```python
from build123d import *

# Parameters (mm, degrees)
BOSS_EXTRU_1_DEPTH      = 5
ESQUISSE2_W             = 17
ESQUISSE2_H             = 18
ENL_V_MAT_EXTRU_1_DEPTH = 253.408894455
ESQUISSE3_W             = 6
ESQUISSE3_H             = 41
BOSS_EXTRU_2_DEPTH      = 70
ENL_V_MAT_EXTRU_3_DEPTH = 223.904127373
CHANFREIN1_SIZE         = 3
ESQUISSE7_R             = 1.5
ENL_V_MAT_EXTRU_4_DEPTH = 25


# Read off the part's stored shape, not the designer's step: Boss.-Extru.1
with BuildPart() as part:
    # Boss.-Extru.1 outline → Boss.-Extru.1 (new body)
    with BuildSketch(Plane.XY):
        Polygon((0, 25.5), (0, 0), (240, 0), (240, 25.5), (245, 25.5), (245, 40.5), (240, 40.5), (240, 60.5), (122.5, 60.5), (122.5, 39.5), (117.5, 39.5), (117.5, 60.5), (0, 60.5), (0, 40.5), (-5, 40.5), (-5, 25.5), align=None)
    extrude(amount=BOSS_EXTRU_1_DEPTH)

    # Esquisse2 → Enlèv. mat.-Extru.1 (cut, through all)
    with BuildSketch(Plane.XY.offset(5)):
        with Locations((231.5, 9)):
            Rectangle(ESQUISSE2_W, ESQUISSE2_H)
        with Locations((8.5, 9)):
            Rectangle(ESQUISSE2_W, ESQUISSE2_H)
    extrude(amount=-ENL_V_MAT_EXTRU_1_DEPTH, mode=Mode.SUBTRACT)

    # Esquisse3 → Boss.-Extru.2 (add)
    with BuildSketch(Plane.XY.offset(5)):
        with Locations((47, 22.5)):
            Rectangle(ESQUISSE3_W, ESQUISSE3_H)
        with Locations((193, 22.5)):
            Rectangle(ESQUISSE3_W, ESQUISSE3_H)
    extrude(amount=BOSS_EXTRU_2_DEPTH)

    # Esquisse6 → Enlèv. mat.-Extru.3 (cut, through all)
    with BuildSketch(Plane.ZY.offset(-44)):
        Polygon((35, 43), (75, 43), (75, 2), (61, 2), align=None)
    extrude(amount=-ENL_V_MAT_EXTRU_3_DEPTH, mode=Mode.SUBTRACT)

    # Chanfrein1
    chanfrein1_edges = [part.edges().sort_by_distance(p)[0] for p in [
        (120, 0, 0),
    ]]
    chamfer(chanfrein1_edges, length=CHANFREIN1_SIZE)

    # Esquisse7 → Enlèv. mat.-Extru.4 (cut)
    with BuildSketch(Plane.XZ.offset(-2)):
        with Locations(Location((47, 25, 0), (0, 0, 270))):
            Circle(ESQUISSE7_R)
        with Locations(Location((47, 41, 0), (0, 0, 270))):
            Circle(ESQUISSE7_R)
        with Locations(Location((193, 41, 0), (0, 0, 270))):
            Circle(ESQUISSE7_R)
        with Locations(Location((193, 25, 0), (0, 0, 270))):
            Circle(ESQUISSE7_R)
    extrude(amount=-ENL_V_MAT_EXTRU_4_DEPTH, mode=Mode.SUBTRACT)


solid = part.part
```
Build history of the part. All positions in model axes, mm. A direction names the side the tool comes from. Round coordinates to 2 decimals unless told otherwise and drop trailing zeros. Write each loop counter-clockwise with the first axis right and the second up, starting at its lowest first coordinate (ties: lowest second). Pieces come first, ordered by that corner, then holes. Notation, with made-up numbers: (8.5, 39) - (47.5, 39) arc R26 cw to (47.5, 77) - close; hole circle Ø2 at (69, 60.5). An arc over 180 degrees is marked (long way). Answer as CSV lines item,"result".
Q1. Cut at C-C (y = 9). Write the cut outline in (x, z), and give its area (3 significant figures).
Report:
outline,"(17, 0) - (223, 0) - (223, 5) - (196, 5) - (196, 56.56) - (190, 56.56) - (190, 5) - (50, 5) - (50, 56.56) - (44, 56.56) - (44, 5) - (17, 5) - close; hole circle Ø3 at (47, 25); hole circle Ø3 at (47, 41); hole circle Ø3 at (193, 25); hole circle Ø3 at (193, 41)"
area,"1,620 mm^2"
Q2. Tool access for faces 1 (the flat face through (231, 18, 3)), 2 (the flat face through (44, 22, 26)), 3 (the flat face through (120, 39.5, 2)), 4 (the flat face through (193, 43, 20)): list every direction of +Z, -Z, +X, -X, +Y, -Y with a clear straight run to the whole face (end or side of a thin tool).
Report:
face 1,"+Z, -Z, +X, -Y"
face 2,"+Z, -X, +Y, -Y"
face 3,"+Z, -Z, +Y"
face 4,"+Z, +X, -X, +Y"
Q3. Drop flat-ended pins along their axis: pin 1 (3 mm diameter, centred on x = 48.5, z = 26, fed in from +Y); pin 2 (2.5 mm diameter, centred on x = 193, z = 41, fed in from +Y); pin 3 (2.5 mm diameter, centred on y = 52, z = 3.5, fed in from -X). Give the stop position or say it passes through.
Report:
pin 1,"stops at y = 43"
pin 2,"stops at y = 35.51"
pin 3,"stops at x = 0"
Q4. Drill centre lines: probe 1 along X at (y, z) = (14, 25); probe 2 along X at (y, z) = (3, 55.5); probe 3 along Z at (x, y) = (193, 12). Where is each one in solid material? Low to high. Write a range as [from, to].
Report:
probe 1,"x = [44, 45.5], [48.5, 50], [190, 191.5], [194.5, 196]"
probe 2,"x = [44, 50], [190, 196]"
probe 3,"z = [0, 23.5], [26.5, 39.5], [42.5, 54.66]"
Q5. Cut at D-D (x = 136.5). Write the cut outline in (y, z).
Report:
outline,"(0, 3) - (3, 0) - (60.5, 0) - (60.5, 5) - (0, 5) - close"
Q6. Pull direction X, two halves, no side cores. Call faces 5 (the flat face through (190, 22, 26)), 6 (the flat face through (193, 2, 33)), 7 (the flat face through (-5, 33, 2)): +X half, -X half, draft (parallel to the pull), parting line (faces both ways), or undercut.
Report:
face 5,"undercut"
face 6,"draft"
face 7,"-X half"
Q7. Cut at B-B (y = 32). Write the cut outline in (x, z).
Report:
outline,"(-5, 0) - (245, 0) - (245, 5) - (196, 5) - (196, 41.98) - (190, 41.98) - (190, 5) - (50, 5) - (50, 41.98) - (44, 41.98) - (44, 5) - (-5, 5) - close"
Q8. Cut at A-A (z = 19.5). Write the cut outline in (x, y), and give its area (3 significant figures).
Report:
outline,"(44, 2) - (50, 2) - (50, 43) - (44, 43) - close; (190, 2) - (196, 2) - (196, 43) - (190, 43) - close"
area,"492 mm^2"
